```python
from build123d import *

# Parameters (mm, degrees)
SKETCH3_R           = 11.43
SKETCH3_R_2         = 8.255
BOSS_EXTRUDE3_DEPTH = 2.54


with BuildPart() as part:
    # Sketch1 → Revolve1 (revolve)
    with BuildSketch(Plane.XY, mode=Mode.PRIVATE) as revolve1_sk:
        with BuildLine():
            Line((-8.255, 16.035758426), (-14.45622882, 16.035758426))
            ThreePointArc((-14.45622882, 16.035758426), (-21.473034234, 2.244304079), (-17.459613398, -12.7))
            Line((-17.459613398, -12.7), (-11.43, -12.7))
            Line((-11.43, -12.7), (-11.43, 8.415758426))
            Line((-11.43, 8.415758426), (-8.255, 8.415758426))
            Line((-8.255, 8.415758426), (-8.255, 16.035758426))
        make_face()
    revolve(revolve1_sk.sketch.rotate(Axis((0, 0, 0), (0, 1, 0)), 180), axis=Axis((0, 0, 0), (0, 1, 0)))

    # Sketch3 → Boss-Extrude3 (add)
    with BuildSketch(Plane.XZ.offset(-8.415758426)):
        Circle(SKETCH3_R)
        Circle(SKETCH3_R_2, mode=Mode.SUBTRACT)
    extrude(amount=BOSS_EXTRUDE3_DEPTH)


solid = part.part
```
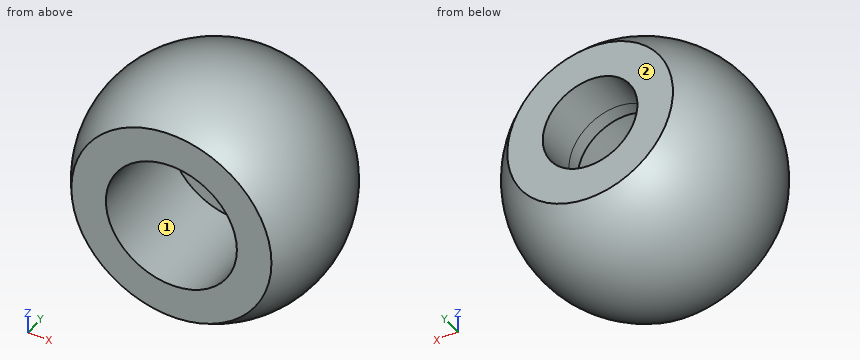
Source: CAD feature listing. Evaluate the final solid. Frame: model axes, mm. Face numbers are marked on the shaded views. Coordinates: 2 decimals unless noted, no trailing zeros. Loops run counter-clockwise (first coordinate to the right, second up) from the corner with the lowest first, then second, coordinate; pieces in that order, holes last. Notation, with made-up numbers: (-33.5, 49.25) -> (4.5, 49.25) arc R19 cw to (4.5, 64.25) -> close; hole circle Ø4 at (79, -30). An arc over 180 degrees is marked (long way). One line per item, written item: value. Start each with the question number.
Q1. Mould query, pull axis X, two halves, no side actions, for the marked faces 1 and 2. Classes: pulls with the +X half, pulls with the -X half, needs draft (parallel to the pull), parting line crosses it, or undercut.
Q2. Section query A-A, the plane x = 0. Return the cut outline in (y, z) (3 decimals), and give its area (3 significant figures).
Q3. Line query: line 1 along Z through (x, y) = (0, -0.25); line 2 along Z through (x, y) = (1.5, 12.75); line 3 along X through (y, z) = (6.5, 3). Output: solid intervals per line, ascending.
Q4. Contact query for flat-ended pins moving along their axis: P1, Ø4, axis at x = 5.5, z = -16.5, coming from the +Y side; P2, Ø1.5, axis at x = -0.5, y = -2, coming from the +Z side; P3, Ø3, axis at y = -5.5, z = 14.5, coming from the -X side. Output: stop coordinate, or through.
Q5. Section query D-D, the plane y = -3.5. Return the cut outline in (x, z), and give its area (3 significant figures).
Q6. Section query B-B, the plane z = 0. Return the cut outline in (x, y) (3 decimals), and give its area (3 significant figures).
Q7. Section query C-C, the plane x = -10.5. Return the cut outline in (y, z).
Results:
1. face 1: undercut
1. face 2: needs draft
2. outline: (-12.7, -17.46) arc R21.59 ccw to (16.036, -14.456) -> (16.036, -8.255) -> (5.876, -8.255) -> (5.876, -11.43) -> (-12.7, -11.43) -> close; (-12.7, 11.43) -> (5.876, 11.43) -> (5.876, 8.255) -> (16.036, 8.255) -> (16.036, 14.456) arc R21.59 ccw to (-12.7, 17.46) -> close
2. area: 545 mm^2
3. line 1: -21.59 to -11.43, 11.43 to 21.59
3. line 2: -17.36 to -8.12, 8.12 to 17.36
3. line 3: -20.37 to -7.69, 7.69 to 20.37
4. P1: y = 15.14
4. P2: z = 21.55
4. P3: x = -16.43
5. outline: circle Ø42.61 at (0, 0); hole circle Ø22.86 at (0, 0)
5. area: 1,020 mm^2
6. outline: (-17.46, -12.7) -> (-11.43, -12.7) -> (-11.43, 5.876) -> (-8.255, 5.876) -> (-8.255, 16.036) -> (-14.456, 16.036) arc R21.59 ccw to start; (8.255, 5.876) -> (11.43, 5.876) -> (11.43, -12.7) -> (17.46, -12.7) arc R21.59 ccw to (14.456, 16.036) -> (8.255, 16.036) -> close
6. area: 545 mm^2
7. outline: (-12.7, -13.95) arc R18.86 ccw to (16.04, -9.94) -> (16.04, 9.94) arc R18.86 ccw to (-12.7, 13.95) -> (-12.7, 4.52) -> (5.88, 4.52) -> (5.88, -4.52) -> (-12.7, -4.52) -> close
